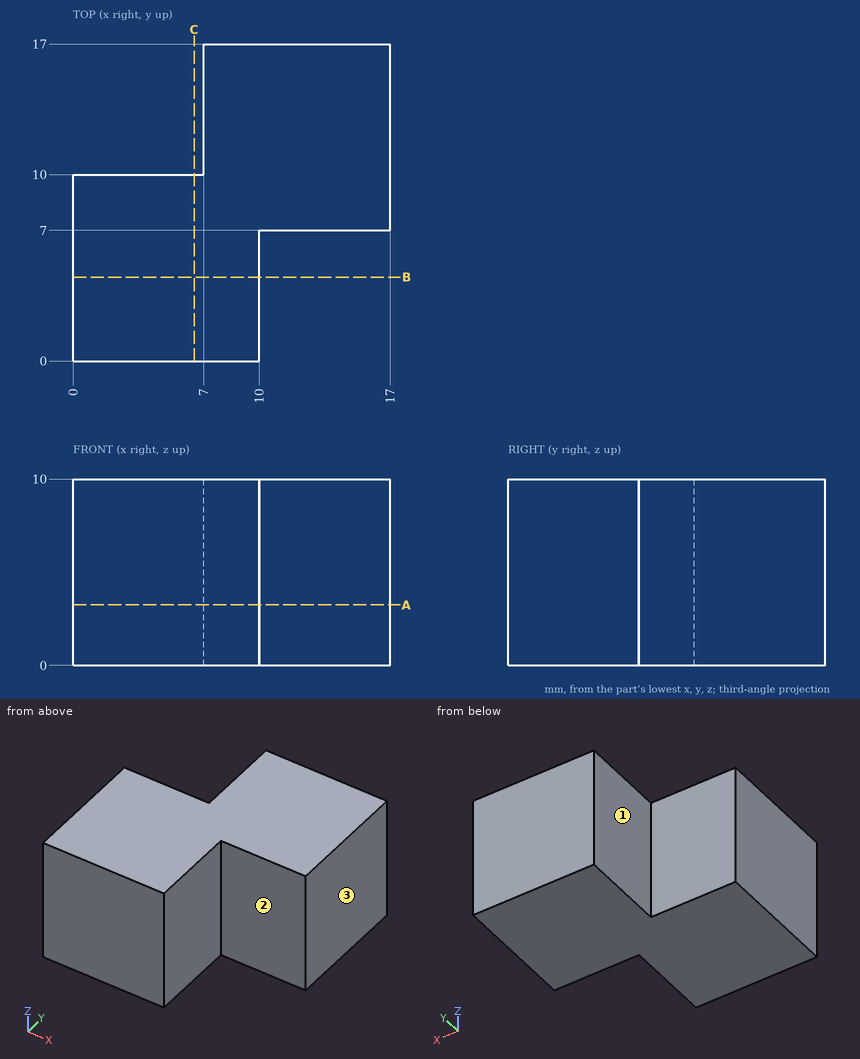
Geometry check sheet. Reference: drawing and pictorial views, mm from the part's lowest x, y, z. A direction names the side the tool comes from. Give positions to 0.01 mm unless a question says otherwise; leave off trailing zeros. Write each loop counter-clockwise with the first axis right and the second up, starting at its lowest first coordinate (ties: lowest second). Pieces come first, ordered by that corner, then holes. Notation, with made-up numbers: (85.25, -37.5) -> (128.25, -37.5) arc R16 ccw to (128.25, -10.5) -> close; hole circle Ø8 at (60.5, 13). An arc over 180 degrees is marked (long way). One line per question, with ' | ' between items.
Item 1: Depth check by flat-ended pin: pin 1 (3.5 mm diameter, centred on y = 4, z = 4, fed in from +X); pin 2 (6 mm diameter, centred on x = 2.5, z = 1, fed in from +Y); pin 3 (2 mm diameter, centred on y = 12, z = 3, fed in from -X). Enter the tip coordinate at first touch or a pass-through.
Determined:
pin 1: x = 10 | pin 2: y = 10 | pin 3: x = 7
Item 2: Access from +Z, -Z, +X, -X, +Y, -Y to the whole of each face (thin tool, end or side, straight path). Record for the marked faces 1, 2 and 3.
Determined:
face 1: +Z, -Z, -X, +Y | face 2: +Z, -Z, +X, -Y | face 3: +Z, -Z, +X, +Y, -Y
Item 3: Sectioned sample at A-A, the plane z = 3.25. Record the boundary of the cut face in (x, y).
Determined:
outline: (0, 0) -> (10, 0) -> (10, 7) -> (17, 7) -> (17, 17) -> (7, 17) -> (7, 10) -> (0, 10) -> close
Item 4: Scan lines: line 1 along X through (y, z) = (10.75, 9); line 2 along X through (y, z) = (1.25, 9). Record each from-to range of solid material in increasing order.
Determined:
line 1: 7 to 17 | line 2: 0 to 10
Item 5: Sectioned sample at B-B, the plane y = 4.5. Record the boundary of the cut face in (x, z), plus the area to 3 significant figures.
Determined:
outline: (0, 0) -> (10, 0) -> (10, 10) -> (0, 10) -> close | area: 100 mm^2
